Model file for the job. Use its own axes, mm. Face numbers are marked on the shaded views. A direction names the side the tool comes from. Round coordinates to 2 decimals unless told otherwise and drop trailing zeros. Loops run counter-clockwise (first coordinate to the right, second up) from the corner with the lowest first, then second, coordinate; pieces in that order, holes last. Notation, with made-up numbers: (58.5, -13) - (84.5, -13) arc R22 ccw to (84.5, 23) - close; hole circle Ø7 at (57, 47.25). An arc over 180 degrees is marked (long way). Answer as a JSON object with one key per item and string values.
Autodesk Inventor part; units mm, degrees
ref_plane "YZ Plane" through (0, 0, 0) normal (1, 0, 0) x (0, 1, 0)
ref_plane "XZ Plane" through (0, 0, 0) normal (0, 1, 0) x (-1, 0, 0)
ref_plane "XY Plane" through (0, 0, 0) normal (0, 0, 1) x (1, 0, 0)
sketch "Эскиз1" plane through (0, 0, 0) normal (0, 0, 1) x (1, 0, 0)
  line L0 (0, 0) -> (20.5, 0)
  line L1 (20.5, 0) -> (20.5, 1.5)
  line L2 (20.5, 1.5) -> (17, 5)
  line L3 (0, 80) -> (3, 80)
  line L4 (17, 5) -> (11, 5)
  arc A0 (3, 13) -> (11, 5) centre (11, 13) ccw
  line L5 (3, 80) -> (3, 76)
  line L6 (3, 76) -> (2.5, 76)
  line L7 (2.5, 76) -> (2.5, 74)
  line L8 (2.5, 74) -> (3, 74)
  line L9 (3, 80) -> (3, 76)
  line L10 (3, 74) -> (3, 13)
  line L11 (0, 80) -> (0, 0)
  dimension "d0" = 20.5
  dimension "d1" = 1.5
  dimension "d2" = 45
  dimension "d3" = 17
  dimension "d4" = 3
  dimension "d5" = 8
  dimension "d6" = 80
  dimension "d7" = 4
  dimension "d8" = 2
  dimension "d9" = 0.5
revolve "Вращение1" add sketch "Эскиз1" angle 360 about axis through (0, 80, 0) along (0, -1, 0)
properties part number "впускной клапан"
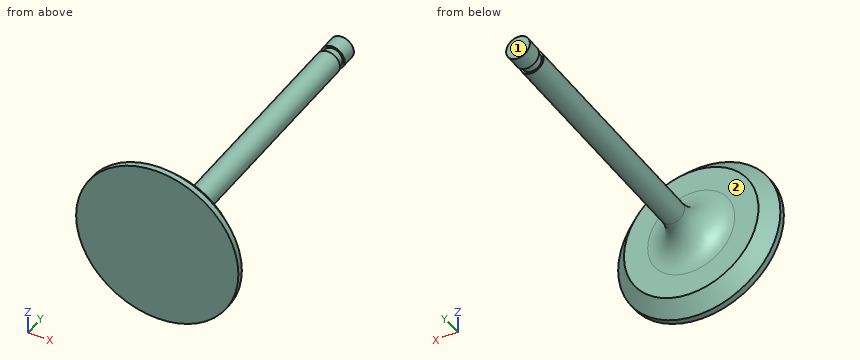
1) Slice it at A-A on z = 0. List the corners of the cut face in (x, y).
Values follow:
{"outline": "(-20.5, 0) - (20.5, 0) - (20.5, 1.5) - (17, 5) - (11, 5) arc R8 cw to (3, 13) - (3, 74) - (2.5, 74) - (2.5, 76) - (3, 76) - (3, 80) - (-3, 80) - (-3, 76) - (-2.5, 76) - (-2.5, 74) - (-3, 74) - (-3, 13) arc R8 cw to (-11, 5) - (-17, 5) - (-20.5, 1.5) - close"}
2) Slice it at C-C on y = 51.5. List the corners of the cut face in (x, z), then the cut area to 3 significant figures.
Values follow:
{"outline": "circle Ø6 at (0, 0)", "area": "28.3 mm²"}
3) Probe probe 1 along Y at (x, z) = (-8, 14.5); probe 2 along Y at (x, z) = (-8.5, -18); probe 3 along X at (y, z) = (40.5, 1). List the from-to ranges inside material, lowest first.
Values follow:
{"probe 1": "0 to 5", "probe 2": "0 to 2.09", "probe 3": "-2.83 to 2.83"}
4) Tool access for the marked faces 1 and 2: list every direction of +Z, -Z, +X, -X, +Y, -Y with a clear straight run to the whole face (end or side of a thin tool).
Values follow:
{"face 1": "+Z, -Z, +X, -X, +Y", "face 2": "+Y"}
5) Slice it at B-B on x = 0. List the corners of the cut face in (y, z), then the cut area to 3 significant figures.
Values follow:
{"outline": "(0, -20.5) - (1.5, -20.5) - (5, -17) - (5, -11) arc R8 cw to (13, -3) - (74, -3) - (74, -2.5) - (76, -2.5) - (76, -3) - (80, -3) - (80, 3) - (76, 3) - (76, 2.5) - (74, 2.5) - (74, 3) - (13, 3) arc R8 cw to (5, 11) - (5, 17) - (1.5, 20.5) - (0, 20.5) - close", "area": "668 mm²"}
6) Drop flat-ended pins along their axis: P1, Ø1.5, axis at x = 8.5, z = -14.5, coming from the +Y side; P2, Ø8, axis at x = -5, y = 26, coming from the -Z side; P3, Ø1, axis at x = 0, y = 57, coming from the -Z side. Give the stop position or say it passes through.
Values follow:
{"P1": "y = 5", "P2": "z = -2.83", "P3": "z = -3"}
